from build123d import *

# Parameters (mm, degrees)
CYLINDER001_R             = 1.5
CYLINDER001_DEPTH         = 23
ARRAY002_X_COUNT          = 2
ARRAY002_X_PITCH          = 10
ARRAY002_Y_COUNT          = 2
ARRAY002_Y_PITCH          = 30
BOX015_W                  = 20
BOX015_H                  = 40
BOX015_DEPTH              = 1.66667
FUSION004_PLACEMENT_ANGLE = 90


with BuildPart() as obj1:
    # Cylinder001 → Cylinder001 (new body)
    with BuildSketch(Plane(origin=(70, 112.5, 0), x_dir=(1, 0, 0), z_dir=(0, 0, 1))):
        Circle(CYLINDER001_R)
    extrude(amount=CYLINDER001_DEPTH)

    # Array002 X: obj1_2


with BuildPart() as obj1_1:
    add(obj1.part)
    with Locations(*[(i * ARRAY002_X_PITCH, 0, 0) for i in range(1, ARRAY002_X_COUNT)]):
        add(obj1.part)

    # Array002 Y: obj1_2


with BuildPart() as obj1_2:
    add(obj1_1.part)
    with Locations(*[(0, i * ARRAY002_Y_PITCH, 0) for i in range(1, ARRAY002_Y_COUNT)]):
        add(obj1_1.part)


with BuildPart() as obj2:
    # Box015 → Box015 (new body)
    with BuildSketch(Plane(origin=(65, 107.5, 23), x_dir=(1, 0, 0), z_dir=(0, 0, 1))):
        with Locations((10, 20)):
            Rectangle(BOX015_W, BOX015_H)
    extrude(amount=BOX015_DEPTH)

    # Fusion004: union obj1
    add(obj1_2.part)


with BuildPart() as obj2_1:
    # Fusion004 placement: moved
    add(obj2.part.moved(Location((210, 0, 97))).rotate(Axis((210, 0, 97), (0, 0, 1)), FUSION004_PLACEMENT_ANGLE))


solid = obj2_1.part
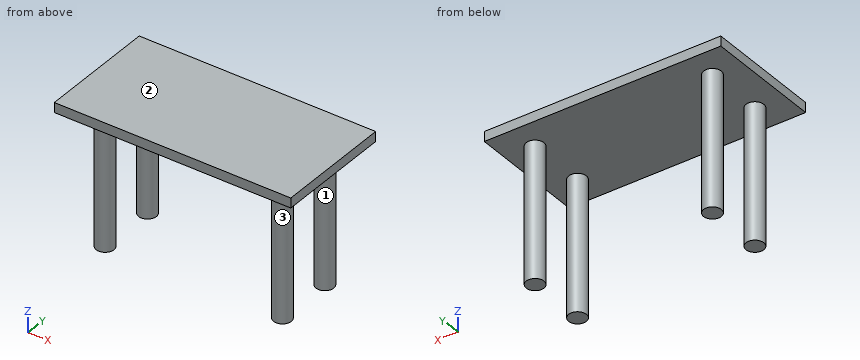
Design review of the part built by this model. Coordinates are the model's own, in mm. Face numbers are marked on the shaded views. Give positions to 0.01 mm unless a question says otherwise; leave off trailing zeros. Loops run counter-clockwise (first coordinate to the right, second up) from the corner with the lowest first, then second, coordinate; pieces in that order, holes last. Notation, with made-up numbers: M 80.25,-2 L 118.25,-2 A14 ccw 118.25,10 Z; hole C 27,60 d1. An arc over 180 degrees is marked long. Answer as a JSON object with one key per item and string values.
Item 1: We need section C-C (z = 101.5). State the section outline as (x, y) points, and give its area (3 significant figures).
Output values:
{"outline": "C 67.5,70 d3; C 67.5,80 d3; C 97.5,70 d3; C 97.5,80 d3", "area": "28.3 mm2"}
Item 2: We need section A-A (x = 97.5). State the section outline as (y, z) points, and give its area (3 significant figures).
Output values:
{"outline": "M 65,120 L 68.5,120 L 68.5,97 L 71.5,97 L 71.5,120 L 78.5,120 L 78.5,97 L 81.5,97 L 81.5,120 L 85,120 L 85,121.67 L 65,121.67 Z", "area": "171 mm2"}
Item 3: Mouldability with a two-part tool opening along Y and no side actions: class the marked faces 1, 2 and 3 as pulls with the +Y half, pulls with the -Y half, needs draft (parallel to the pull), parting line crosses it, or undercut.
Output values:
{"face 1": "undercut", "face 2": "needs draft", "face 3": "undercut"}
Item 4: Wall thickness on line 1 along Z through (x, y) = (79, 83.5); line 2 along X through (y, z) = (68.75, 116); line 3 along X through (y, z) = (80.25, 103.5): over which ranges is each line inside the solid? List them lowest first.
Output values:
{"line 1": "z = 120 to 121.67", "line 2": "x = 66.67 to 68.33, 96.67 to 98.33", "line 3": "x = 66.02 to 68.98, 96.02 to 98.98"}
Item 5: For P1, Ø8, axis at x = 74.5, y = 77.5, coming from the -Z side; P2, Ø6, axis at y = 79, z = 101.5, coming from the -X side; P3, Ø2, axis at y = 81.5, z = 110, coming from the -X side, all flat-tipped, find the tip position at first contact; note any pin that passes through.
Output values:
{"P1": "stops at z = 120", "P2": "stops at x = 66", "P3": "stops at x = 66.09"}
Item 6: We need section B-B (y = 70). State the section outline as (x, z) points.
Output values:
{"outline": "M 62.5,120 L 66,120 L 66,97 L 69,97 L 69,120 L 96,120 L 96,97 L 99,97 L 99,120 L 102.5,120 L 102.5,121.67 L 62.5,121.67 Z"}
Item 7: We need section D-D (y = 75). State the section outline as (x, z) points.
Output values:
{"outline": "M 62.5,120 L 102.5,120 L 102.5,121.67 L 62.5,121.67 Z"}
